Can you work these out from the drawing? Everything is in mm from the part's minimum corner. A direction names the side the tool comes from. Coordinates: 2 decimals unless noted, no trailing zeros. Loops run counter-clockwise (first coordinate to the right, second up) from the corner with the lowest first, then second, coordinate; pieces in that order, holes last. Notation, with made-up numbers: (53.5, -10) - (99.5, -10) arc R8 cw to (99.5, 3) - close; hole circle Ø10 at (44.5, 13.25). An arc over 180 degrees is marked (long way). Use CSV: the item, a comma, the result in double quotes.
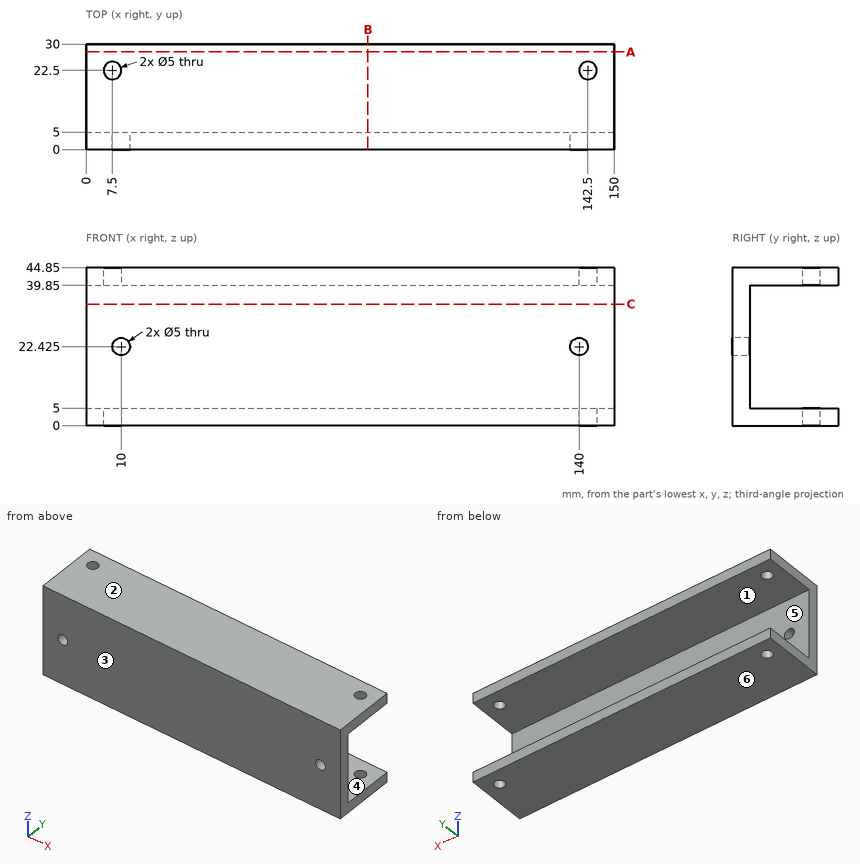
(1) Suppose I cut it at C-C (z = 34.5). Write out the boundary of the cut face in (x, y), plus the area to 3 significant figures.
Computed:
outline,"(0, 0) - (150, 0) - (150, 5) - (0, 5) - close"
area,"750 mm²"
(2) Suppose I cut it at A-A (y = 27.75). Write out the boundary of the cut face in (x, z), plus the area to 3 significant figures.
Computed:
outline,"(0, 0) - (150, 0) - (150, 5) - (0, 5) - close; (0, 39.85) - (150, 39.85) - (150, 44.85) - (0, 44.85) - close"
area,"1,500 mm²"
(3) Suppose I cut it at B-B (x = 80). Write out the boundary of the cut face in (y, z).
Computed:
outline,"(0, 0) - (30, 0) - (30, 5) - (5, 5) - (5, 39.85) - (30, 39.85) - (30, 44.85) - (0, 44.85) - close"
(4) Which directions (+Z, -Z, +X, -X, +Y, -Y) give clear straight access to the entire face, cutting with the end or side of a thin tool? Please do the marked faces 5 and 6.
Computed:
face 5,"+X, -X, +Y"
face 6,"-Z, +X, -X, +Y, -Y"
(5) Will these pins go through, and if not, where does the flat tip stop? pin 1 (6 mm diameter, centred on x = 142.5, y = 22.5, fed in from -Z); pin 2 (6 mm diameter, centred on x = 112.5, z = 17.5, fed in from +Y); pin 3 (5 mm diameter, centred on y = 9.5, z = 11.5, fed in from +X).
Computed:
pin 1,"stops at z = 0"
pin 2,"stops at y = 5"
pin 3,"passes through"
(6) Please list where these lines run through material, in increasing order: line 1 (Z direction, x = 140, y = 1.6) (3 decimals); line 2 (Z direction, x = 6, y = 19.5); line 3 (Y direction, x = 142.5, z = 41.4).
Computed:
line 1,"z = 0 to 19.925, 24.925 to 44.85"
line 2,"z = 0 to 5, 39.85 to 44.85"
line 3,"y = 0 to 20, 25 to 30"
(7) Thinking about a two-plate mould opening in Z: for the marked faces 1, 2, 3 and 4, which applies, +Z half, -Z half, draft (parallel to the pull), parting line (faces both ways), or undercut?
Computed:
face 1,"undercut"
face 2,"+Z half"
face 3,"draft"
face 4,"undercut"
